Work out the finished part from the listing and answer in its coordinate system (mm). Round coordinates to 2 decimals unless told otherwise and drop trailing zeros. Order: outer loops, then holes, each group sorted by start corner. A loop starts at its lowest first (then second) coordinate and runs counter-clockwise, first axis right, second up.
from build123d import *

# Parameters (mm, degrees)
SKETCH1_R           = 28.645714286
SKETCH1_R_2         = 23.645714286
BOSS_EXTRUDE1_DEPTH = 5
SKETCH3_R           = 1.7
CUT_EXTRUDE1_DEPTH  = 8


with BuildPart() as part:
    # Sketch1 → Boss-Extrude1 (new body)
    with BuildSketch(Plane.XY):
        Circle(SKETCH1_R)
        Circle(SKETCH1_R_2, mode=Mode.SUBTRACT)
    extrude(amount=BOSS_EXTRUDE1_DEPTH)

    # Sketch3 → Cut-Extrude1 (cut, symmetric)
    with BuildSketch(Plane.XY.offset(2.5)):
        with Locations((28.645714286, 0)):
            Circle(SKETCH3_R)
        with Locations((28.210521519, -4.974276084)):
            Circle(SKETCH3_R)
        with Locations((26.918166331, -9.797411306)):
            Circle(SKETCH3_R)
        with Locations((24.807916281, -14.322857143)):
            Circle(SKETCH3_R)
        with Locations((21.943890248, -18.413110214)):
            Circle(SKETCH3_R)
        with Locations((18.413110214, -21.943890248)):
            Circle(SKETCH3_R)
        with Locations((14.322857143, -24.807916281)):
            Circle(SKETCH3_R)
        with Locations((9.797411306, -26.918166331)):
            Circle(SKETCH3_R)
        with Locations((4.974276084, -28.210521519)):
            Circle(SKETCH3_R)
        with Locations((0, -28.645714286)):
            Circle(SKETCH3_R)
        with Locations((-4.974276084, -28.210521519)):
            Circle(SKETCH3_R)
        with Locations((-9.797411306, -26.918166331)):
            Circle(SKETCH3_R)
        with Locations((-14.322857143, -24.807916281)):
            Circle(SKETCH3_R)
        with Locations((-18.413110214, -21.943890248)):
            Circle(SKETCH3_R)
        with Locations((-21.943890248, -18.413110214)):
            Circle(SKETCH3_R)
        with Locations((-24.807916281, -14.322857143)):
            Circle(SKETCH3_R)
        with Locations((-26.918166331, -9.797411306)):
            Circle(SKETCH3_R)
        with Locations((-28.210521519, -4.974276084)):
            Circle(SKETCH3_R)
        with Locations((-28.645714286, 0)):
            Circle(SKETCH3_R)
        with Locations((-28.210521519, 4.974276084)):
            Circle(SKETCH3_R)
        with Locations((-26.918166331, 9.797411306)):
            Circle(SKETCH3_R)
        with Locations((-24.807916281, 14.322857143)):
            Circle(SKETCH3_R)
        with Locations((-21.943890248, 18.413110214)):
            Circle(SKETCH3_R)
        with Locations((-18.413110214, 21.943890248)):
            Circle(SKETCH3_R)
        with Locations((-14.322857143, 24.807916281)):
            Circle(SKETCH3_R)
        with Locations((-9.797411306, 26.918166331)):
            Circle(SKETCH3_R)
        with Locations((-4.974276084, 28.210521519)):
            Circle(SKETCH3_R)
        with Locations((0, 28.645714286)):
            Circle(SKETCH3_R)
        with Locations((4.974276084, 28.210521519)):
            Circle(SKETCH3_R)
        with Locations((9.797411306, 26.918166331)):
            Circle(SKETCH3_R)
        with Locations((14.322857143, 24.807916281)):
            Circle(SKETCH3_R)
        with Locations((18.413110214, 21.943890248)):
            Circle(SKETCH3_R)
        with Locations((21.943890248, 18.413110214)):
            Circle(SKETCH3_R)
        with Locations((24.807916281, 14.322857143)):
            Circle(SKETCH3_R)
        with Locations((26.918166331, 9.797411306)):
            Circle(SKETCH3_R)
        with Locations((28.210521519, 4.974276084)):
            Circle(SKETCH3_R)
    extrude(amount=CUT_EXTRUDE1_DEPTH, both=True, mode=Mode.SUBTRACT)


solid = part.part
Item 1: Find the intervals of material crossed by line 1 along Y through (x, z) = (0, 1.15); line 2 along Y through (x, z) = (3, 2.2); line 3 along X through (y, z) = (8.5, 1.45), in increasing order.
Item 2: For a pull along Y with two mould halves and no side action, classify faces 1 (the face through (-5.126, -23.083, 2.465)), 2 (the face through (13.5, -23.32, 2.54)), 3 (the face through (28.536, -2.508, 2.465)), 4 (the face through (16.44, 23.46, 2.46)) as released by +Y, released by -Y, zero draft, split by the parting line, or undercut.
Item 3: Given pin 1 (12 mm diameter, centred on x = -20.5, y = 17.5, fed in from -Z); pin 2 (2 mm diameter, centred on y = -18.5, z = 3.5, fed in from -X), each flat-ended and moving along its own axis, determine where each tip first touches the part or whether it passes through.
Item 4: Find section A-A (y = 0). Write down the section's boundary in (x, z), plus the area to 3 significant figures.
Model answer:
1. line 1: y = -26.95 to -23.65, 23.65 to 26.95
1. line 2: y = -28.49 to -23.45, 23.45 to 28.49
1. line 3: x = -25.82 to -22.07, 22.07 to 25.82
2. face 1: undercut
2. face 2: undercut
2. face 3: released by -Y
2. face 4: released by +Y
3. pin 1: stops at z = 0
3. pin 2: stops at x = -20.64
4. outline: (-26.95, 0) - (-23.65, 0) - (-23.65, 5) - (-26.95, 5) - close; (23.65, 0) - (26.95, 0) - (26.95, 5) - (23.65, 5) - close
4. area: 33.0 mm2
